```python
from build123d import *

# Parameters (mm, degrees)
SKETCH1_R           = 2.54
BOSS_EXTRUDE1_DEPTH = 5.08
BOSS_EXTRUDE2_DEPTH = 2.54
BOSS_EXTRUDE3_DEPTH = 2.54


with BuildPart() as part:
    # Sketch1 → Boss-Extrude1 (new, symmetric)
    with BuildSketch(Plane.XY):
        Circle(SKETCH1_R)
    extrude(amount=BOSS_EXTRUDE1_DEPTH, both=True)

    # Sketch2 → Boss-Extrude2 (add, symmetric)
    with BuildSketch(Plane.XY):
        with BuildLine():
            Line((2.54, 0), (2.54, 75.586789755))
            ThreePointArc((2.54, 75.586789755), (2.383201592, 75.821455156), (2.106394878, 75.766394878))
            Line((2.106394878, 75.766394878), (-21.675690723, 51.984309277))
            ThreePointArc((-21.675690723, 51.984309277), (-22.367766915, 50.698965368), (-22.237970294, 49.244925735))
            Line((-22.237970294, 49.244925735), (-2.54, 0))
            Line((-2.54, 0), (-2.54, -12.7))
            Line((-2.54, -12.7), (2.54, -12.7))
            Line((2.54, -12.7), (2.54, 0))
        make_face()
    extrude(amount=BOSS_EXTRUDE2_DEPTH, both=True)

    # Sketch3 → Boss-Extrude3 (add, symmetric)
    with BuildSketch(Plane.XY):
        Polygon((2.54, 75.586789755), (3.199911358, 75.205789755), (2.54, 74.824789755), align=None)
        Polygon((2.54, 74.570789755), (3.199911358, 74.189789755), (2.54, 73.808789755), align=None)
        Polygon((2.54, 73.554789755), (3.199911358, 73.173789755), (2.54, 72.792789755), align=None)
        Polygon((2.54, 72.538789755), (3.199911358, 72.157789755), (2.54, 71.776789755), align=None)
        Polygon((2.54, 71.522789755), (3.199911358, 71.141789755), (2.54, 70.760789755), align=None)
        Polygon((2.54, 70.506789755), (3.199911358, 70.125789755), (2.54, 69.744789755), align=None)
        Polygon((2.54, 69.490789755), (3.199911358, 69.109789755), (2.54, 68.728789755), align=None)
        Polygon((2.54, 68.474789755), (3.199911358, 68.093789755), (2.54, 67.712789755), align=None)
        Polygon((2.54, 67.458789755), (3.199911358, 67.077789755), (2.54, 66.696789755), align=None)
        Polygon((2.54, 66.442789755), (3.199911358, 66.061789755), (2.54, 65.680789755), align=None)
        Polygon((2.54, 65.426789755), (3.199911358, 65.045789755), (2.54, 64.664789755), align=None)
        Polygon((2.54, 64.410789755), (3.199911358, 64.029789755), (2.54, 63.648789755), align=None)
        Polygon((2.54, 63.394789755), (3.199911358, 63.013789755), (2.54, 62.632789755), align=None)
        Polygon((2.54, 62.378789755), (3.199911358, 61.997789755), (2.54, 61.616789755), align=None)
        Polygon((2.54, 61.362789755), (3.199911358, 60.981789755), (2.54, 60.600789755), align=None)
        Polygon((2.54, 60.346789755), (3.199911358, 59.965789755), (2.54, 59.584789755), align=None)
        Polygon((2.54, 59.330789755), (3.199911358, 58.949789755), (2.54, 58.568789755), align=None)
        Polygon((2.54, 58.314789755), (3.199911358, 57.933789755), (2.54, 57.552789755), align=None)
        Polygon((2.54, 57.298789755), (3.199911358, 56.917789755), (2.54, 56.536789755), align=None)
        Polygon((2.54, 56.282789755), (3.199911358, 55.901789755), (2.54, 55.520789755), align=None)
        Polygon((2.54, 55.266789755), (3.199911358, 54.885789755), (2.54, 54.504789755), align=None)
        Polygon((2.54, 54.250789755), (3.199911358, 53.869789755), (2.54, 53.488789755), align=None)
        Polygon((2.54, 53.234789755), (3.199911358, 52.853789755), (2.54, 52.472789755), align=None)
        Polygon((2.54, 52.218789755), (3.199911358, 51.837789755), (2.54, 51.456789755), align=None)
        Polygon((2.54, 51.202789755), (3.199911358, 50.821789755), (2.54, 50.440789755), align=None)
        Polygon((2.54, 50.186789755), (3.199911358, 49.805789755), (2.54, 49.424789755), align=None)
        Polygon((2.54, 49.170789755), (3.199911358, 48.789789755), (2.54, 48.408789755), align=None)
        Polygon((2.54, 48.154789755), (3.199911358, 47.773789755), (2.54, 47.392789755), align=None)
        Polygon((2.54, 47.138789755), (3.199911358, 46.757789755), (2.54, 46.376789755), align=None)
        Polygon((2.54, 46.122789755), (3.199911358, 45.741789755), (2.54, 45.360789755), align=None)
        Polygon((2.54, 45.106789755), (3.199911358, 44.725789755), (2.54, 44.344789755), align=None)
        Polygon((2.54, 44.090789755), (3.199911358, 43.709789755), (2.54, 43.328789755), align=None)
        Polygon((2.54, 43.074789755), (3.199911358, 42.693789755), (2.54, 42.312789755), align=None)
        Polygon((2.54, 42.058789755), (3.199911358, 41.677789755), (2.54, 41.296789755), align=None)
        Polygon((2.54, 41.042789755), (3.199911358, 40.661789755), (2.54, 40.280789755), align=None)
        Polygon((2.54, 40.026789755), (3.199911358, 39.645789755), (2.54, 39.264789755), align=None)
        Polygon((2.54, 39.010789755), (3.199911358, 38.629789755), (2.54, 38.248789755), align=None)
        Polygon((2.54, 37.994789755), (3.199911358, 37.613789755), (2.54, 37.232789755), align=None)
        Polygon((2.54, 36.978789755), (3.199911358, 36.597789755), (2.54, 36.216789755), align=None)
        Polygon((2.54, 35.962789755), (3.199911358, 35.581789755), (2.54, 35.200789755), align=None)
        Polygon((2.54, 34.946789755), (3.199911358, 34.565789755), (2.54, 34.184789755), align=None)
        Polygon((2.54, 33.930789755), (3.199911358, 33.549789755), (2.54, 33.168789755), align=None)
        Polygon((2.54, 32.914789755), (3.199911358, 32.533789755), (2.54, 32.152789755), align=None)
        Polygon((2.54, 31.898789755), (3.199911358, 31.517789755), (2.54, 31.136789755), align=None)
        Polygon((2.54, 30.882789755), (3.199911358, 30.501789755), (2.54, 30.120789755), align=None)
        Polygon((2.54, 29.866789755), (3.199911358, 29.485789755), (2.54, 29.104789755), align=None)
        Polygon((2.54, 28.850789755), (3.199911358, 28.469789755), (2.54, 28.088789755), align=None)
        Polygon((2.54, 27.834789755), (3.199911358, 27.453789755), (2.54, 27.072789755), align=None)
        Polygon((2.54, 26.818789755), (3.199911358, 26.437789755), (2.54, 26.056789755), align=None)
        Polygon((2.54, 25.802789755), (3.199911358, 25.421789755), (2.54, 25.040789755), align=None)
        Polygon((2.54, 24.786789755), (3.199911358, 24.405789755), (2.54, 24.024789755), align=None)
        Polygon((2.54, 23.770789755), (3.199911358, 23.389789755), (2.54, 23.008789755), align=None)
        Polygon((2.54, 22.754789755), (3.199911358, 22.373789755), (2.54, 21.992789755), align=None)
        Polygon((2.54, 21.738789755), (3.199911358, 21.357789755), (2.54, 20.976789755), align=None)
        Polygon((2.54, 20.722789755), (3.199911358, 20.341789755), (2.54, 19.960789755), align=None)
        Polygon((2.54, 19.706789755), (3.199911358, 19.325789755), (2.54, 18.944789755), align=None)
        Polygon((2.54, 18.690789755), (3.199911358, 18.309789755), (2.54, 17.928789755), align=None)
    extrude(amount=BOSS_EXTRUDE3_DEPTH, both=True)


solid = part.part
```
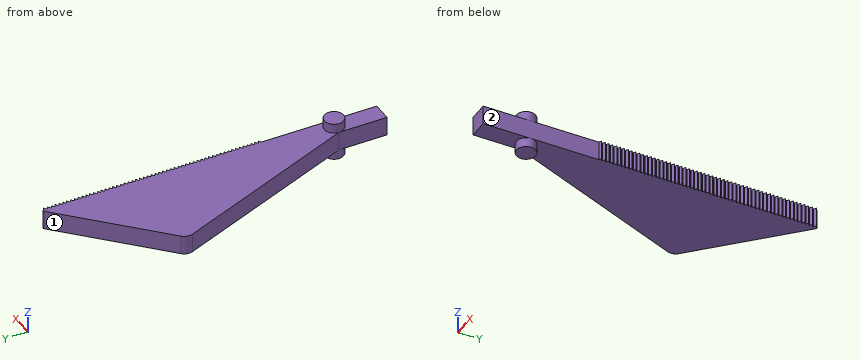
The model under review builds one solid part; all positions refer to its coordinate system, in mm. Face numbers are marked on the shaded views. Give positions to 0.01 mm unless a question says otherwise; leave off trailing zeros. Write each loop counter-clockwise with the first axis right and the second up, starting at its lowest first coordinate (ties: lowest second). Pieces come first, ordered by that corner, then holes. Notation, with made-up numbers: (-21, -0.75) - (17, -0.75) arc R12 ccw to (17, 16.25) - close; hole circle Ø11 at (-28, 49.25). An arc over 180 degrees is marked (long way). Answer in a Markdown table with one row per item. Add a question column.
1. We need section B-B on y = 12. Write out the cut boundary in (x, z).
2. Draft analysis for pull direction Y (two halves, no side actions). For the marked faces 1 and 2, state which applies: +Y half, -Y half, draft (parallel to the pull), parting line (faces both ways), or undercut.
3. Insertion check: P1, Ø5.5, axis at x = 0.5, y = -7.5, coming from the +Z side; P2, Ø6, axis at y = 23, z = 0.5, coming from the -X side; P3, Ø2, axis at x = -13, z = 2, coming from the -Y side. Each pin has a flat end and moves straight along its axis. Give the tip position at first contact, or say it passes through.
4. We need section C-C on x = -13.5. Write out the cut boundary in (y, z).
5. We need section A-A on x = 0. Write out the cut boundary in (y, z).
6. Wall thickness on line 1 along Y through (x, z) = (-0.5, -1); line 2 along Z through (x, y) = (-2.75, 50.5); line 3 along Y through (x, z) = (2.25, 1.25): over which ranges is each line inside the solid? List them lowest first. Write a range as [from, to].
Ans:
| question | item | result |
|---|---|---|
| 1 | outline | (-7.34, -2.54) - (2.54, -2.54) - (2.54, 2.54) - (-7.34, 2.54) - close |
| 2 | face 1 | +Y half |
| 2 | face 2 | draft |
| 3 | P1 | stops at z = 2.54 |
| 3 | P2 | stops at x = -12.94 |
| 3 | P3 | stops at y = 23.65 |
| 4 | outline | (27.4, -2.54) - (60.16, -2.54) - (60.16, 2.54) - (27.4, 2.54) - close |
| 5 | outline | (-12.7, -2.54) - (-2.54, -2.54) - (-2.54, -5.08) - (2.54, -5.08) - (2.54, -2.54) - (73.66, -2.54) - (73.66, 2.54) - (2.54, 2.54) - (2.54, 5.08) - (-2.54, 5.08) - (-2.54, 2.54) - (-12.7, 2.54) - close |
| 6 | line 1 | y = [-12.7, 73.16] |
| 6 | line 2 | z = [-2.54, 2.54] |
| 6 | line 3 | y = [-12.7, 75.84] |
